```python
from build123d import *

# Parameters (mm, degrees)
SKETCH1_W            = 500
SKETCH1_H            = 341.5
BOSS_EXTRUDE1_DEPTH  = 12
SKETCH5_W            = 12
SKETCH5_H            = 80
CUT_EXTRUDE2_DEPTH   = 606.612293468
SKETCH3_W            = 441.52
SKETCH3_H            = 278
CUT_EXTRUDE3_DEPTH   = 606.612293468
SKETCH6_W            = 154.666666667
SKETCH6_H            = 12
CUT_EXTRUDE4_DEPTH   = 606.612293468
SCALE1_SCALE         = 0.5
M3_CLEARANCE_SLOT1_D = 3.2
M3_CLEARANCE_SLOT2_D = 3.2


with BuildPart() as part:
    # Sketch1 → Boss-Extrude1 (new body)
    with BuildSketch(Plane.XY):
        with Locations((250, 170.75)):
            Rectangle(SKETCH1_W, SKETCH1_H)
    extrude(amount=BOSS_EXTRUDE1_DEPTH)

    # Sketch5 → Cut-Extrude2 (cut, through all)
    with BuildSketch(Plane.XY.offset(12)):
        with Locations((6, 301.5)):
            Rectangle(SKETCH5_W, SKETCH5_H)
        with Locations((6, 40)):
            Rectangle(SKETCH5_W, SKETCH5_H)
        with Locations((494, 301.5)):
            Rectangle(SKETCH5_W, SKETCH5_H)
        with Locations((494, 40)):
            Rectangle(SKETCH5_W, SKETCH5_H)
    extrude(amount=-CUT_EXTRUDE2_DEPTH, mode=Mode.SUBTRACT)

    # Sketch3 → Cut-Extrude3 (cut, through all)
    with BuildSketch(Plane.XY.offset(12)):
        with Locations((250, 170.75)):
            Rectangle(SKETCH3_W, SKETCH3_H)
    extrude(amount=-CUT_EXTRUDE3_DEPTH, mode=Mode.SUBTRACT)

    # Sketch6 → Cut-Extrude4 (cut, through all)
    with BuildSketch(Plane.XY.offset(12)):
        with Locations((410.666666667, 335.5)):
            Rectangle(SKETCH6_W, SKETCH6_H)
        with Locations((89.333333334, 335.5)):
            Rectangle(SKETCH6_W, SKETCH6_H)
    extrude(amount=-CUT_EXTRUDE4_DEPTH, mode=Mode.SUBTRACT)


with BuildPart() as part_1:
    # Scale1: scaled about (250, 155.633318535, 6)
    add(part.part.scale(SCALE1_SCALE).moved(Location((125, 77.816659268, 3))))

    # M3 Clearance Slot1 (through all)
    with Locations(Plane.XY.offset(9)):
        with Locations((219.02, 239.491659268), (303.98, 239.491659268), (224.52, 84.291659268), (285.36, 84.291659268)):
            Hole(M3_CLEARANCE_SLOT1_D / 2)

    # M3 Clearance Slot2 (through all)
    with Locations(Plane.XY.offset(9)):
        with Locations((254.94, 84.296659268), (254.94, 239.491659268)):
            Hole(M3_CLEARANCE_SLOT2_D / 2)


solid = part_1.part
```
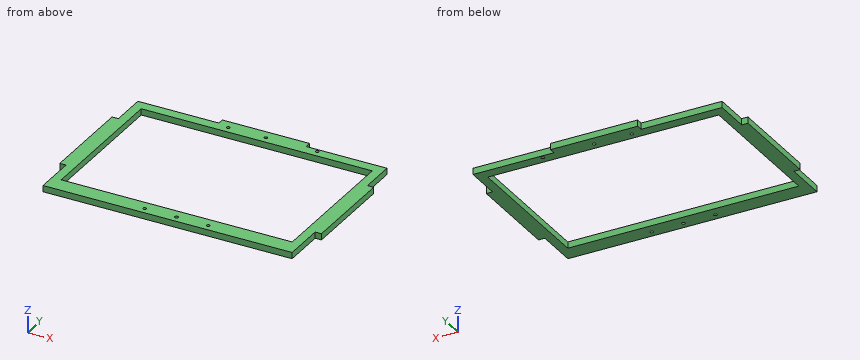
Input: part model. Units: mm. Frame: model coordinates. Coordinates: 2 decimals unless noted, no trailing zeros. Write each loop counter-clockwise with the first axis right and the second up, starting at its lowest first coordinate (ties: lowest second). Pieces come first, ordered by that corner, then holes. Notation, with made-up numbers: (26.5, 47) -> (32.5, 47) arc R19 cw to (32.5, 73) -> close; hole circle Ø10 at (43, 46.25). An arc over 180 degrees is marked (long way). Write each question's results on one line, items separated by ' | '.
Item 1: Section query A-A on y = 138. Return loops of the section in (x, z), plus the area to 3 significant figures.
Conclusion:
outline: (125, 3) -> (139.62, 3) -> (139.62, 9) -> (125, 9) -> close; (360.38, 3) -> (375, 3) -> (375, 9) -> (360.38, 9) -> close | area: 175 mm^2
Item 2: Section query C-C on z = 6.5. Return loops of the section in (x, y), plus the area to 3 significant figures.
Conclusion:
outline: (125, 117.82) -> (131, 117.82) -> (131, 77.82) -> (369, 77.82) -> (369, 117.82) -> (375, 117.82) -> (375, 208.57) -> (369, 208.57) -> (369, 242.57) -> (291.67, 242.57) -> (291.67, 248.57) -> (208.33, 248.57) -> (208.33, 242.57) -> (131, 242.57) -> (131, 208.57) -> (125, 208.57) -> close; hole (139.62, 93.69) -> (360.38, 93.69) -> (360.38, 232.69) -> (139.62, 232.69) -> close; hole circle Ø3.2 at (219.02, 239.49); hole circle Ø3.2 at (224.52, 84.29); hole circle Ø3.2 at (254.94, 84.3); hole circle Ø3.2 at (254.94, 239.49); hole circle Ø3.2 at (285.36, 84.29); hole circle Ø3.2 at (303.98, 239.49) | area: 10,100 mm^2
Item 3: Material intervals for probe 1 along Y at (x, z) = (285.36, 6.75); probe 2 along X at (y, z) = (163, 6.1); probe 3 along Y at (x, z) = (254.94, 7.5), sorted ascending.
Conclusion:
probe 1: y = 77.82 to 82.69, 85.89 to 93.69, 232.69 to 248.57 | probe 2: x = 125 to 139.62, 360.38 to 375 | probe 3: y = 77.82 to 82.7, 85.9 to 93.69, 232.69 to 237.89, 241.09 to 248.57
Item 4: Pin query (flat end, axial travel): pin 1 Ø3 at (y, z) = (97, 5.5) entering from -X; pin 2 Ø3 at (x, z) = (129, 4.5) entering from -Y; pin 3 Ø3 at (y, z) = (247, 6.5) entering from -X; pin 4 Ø2.5 at (x, y) = (219.02, 239.49) entering from +Z. Return the tip coordinate at first contact, or that it passes through.
Conclusion:
pin 1: stops at x = 131 | pin 2: stops at y = 117.82 | pin 3: stops at x = 208.33 | pin 4: passes through
Item 5: Section query B-B on x = 152.5. Return loops of the section in (y, z).
Conclusion:
outline: (77.82, 3) -> (93.69, 3) -> (93.69, 9) -> (77.82, 9) -> close; (232.69, 3) -> (242.57, 3) -> (242.57, 9) -> (232.69, 9) -> close
